from build123d import *

# Parameters (mm, degrees)
SKETCH_1_W          = 250
SKETCH_1_H          = 30
EXTRUDE_1_DEPTH     = 11
SKETCH_4_W          = 15
SKETCH_4_H          = 5
EXTRUDE_2_DEPTH     = 25
CUT_EXTRUDE_2_DEPTH = 251
CUT_EXTRUDE_3_DEPTH = 21
SKETCH_11_W         = 30
SKETCH_11_H         = 10
EXTRUDE_4_DEPTH     = 25
SKETCH_12_R         = 1.6
CUT_EXTRUDE_5_DEPTH = 21
FILLET_1_R          = 10
SKETCH_13_W         = 2
SKETCH_13_H         = 26.2
CUT_EXTRUDE_6_DEPTH = 37
CHAMFER_1_SIZE      = 1


with BuildPart() as part:
    # 草圖1 → 填料-伸長1 (new body)
    with BuildSketch(Plane.XY):
        with Locations((125, 15)):
            Rectangle(SKETCH_1_W, SKETCH_1_H)
    extrude(amount=EXTRUDE_1_DEPTH)

    # 草圖4 → 填料-伸長2 (add)
    with BuildSketch(Plane(origin=(0, 0, 0), x_dir=(-1, 0, 0), z_dir=(0, 0, -1))):
        with Locations((-132.5, 12.5)):
            Rectangle(SKETCH_4_W, SKETCH_4_H)
        with Locations((-132.5, 17.5)):
            Rectangle(SKETCH_4_W, SKETCH_4_H)
        with Locations((-117.5, 17.5)):
            Rectangle(SKETCH_4_W, SKETCH_4_H)
        with Locations((-117.5, 12.5)):
            Rectangle(SKETCH_4_W, SKETCH_4_H)
    extrude(amount=EXTRUDE_2_DEPTH)

    # 草圖5 → 除料-伸長2 (cut, through all)
    with BuildSketch(Plane(origin=(250, 0, 0), x_dir=(0, 0, -1), z_dir=(1, 0, 0))):
        Polygon((-11, 15), (-7, 15), (-7, 18), (-11, 21), align=None)
        Polygon((-7, 12), (-7, 15), (-11, 15), (-11, 9), align=None)
    extrude(amount=-CUT_EXTRUDE_2_DEPTH, mode=Mode.SUBTRACT)

    # 草圖6 → 除料-伸長3 (cut, through all)
    with BuildSketch(Plane.XZ.offset(-10)):
        with BuildLine():
            ThreePointArc((126.6, -12.5), (126.13137085, -11.36862915), (125, -10.9))
            Line((125, -10.9), (125, -12.5))
            Line((125, -12.5), (126.6, -12.5))
        make_face()
        with BuildLine():
            Line((125, -12.5), (125, -10.9))
            ThreePointArc((125, -10.9), (123.86862915, -11.36862915), (123.4, -12.5))
            Line((123.4, -12.5), (125, -12.5))
        make_face()
        with BuildLine():
            Line((126.6, -12.5), (125, -12.5))
            Line((125, -12.5), (125, -14.1))
            ThreePointArc((125, -14.1), (126.13137085, -13.63137085), (126.6, -12.5))
        make_face()
        with BuildLine():
            Line((125, -14.1), (125, -12.5))
            Line((125, -12.5), (123.4, -12.5))
            ThreePointArc((123.4, -12.5), (123.86862915, -13.63137085), (125, -14.1))
        make_face()
    extrude(amount=-CUT_EXTRUDE_3_DEPTH, mode=Mode.SUBTRACT)

    # 草圖11 → 填料-伸長4 (add)
    with BuildSketch(Plane(origin=(0, 0, 0), x_dir=(-1, 0, 0), z_dir=(0, 0, -1))):
        with Locations((-225, 15)):
            Rectangle(SKETCH_11_W, SKETCH_11_H)
    extrude(amount=EXTRUDE_4_DEPTH)

    # 草圖12 → 除料-伸長5 (cut, through all)
    with BuildSketch(Plane(origin=(0, 20, 0), x_dir=(1, 0, 0), z_dir=(0, 1, 0))):
        with Locations((225, 12.5)):
            Circle(SKETCH_12_R)
    extrude(amount=-CUT_EXTRUDE_5_DEPTH, mode=Mode.SUBTRACT)

    # 圓角1
    fillet_1_edges = [part.edges().sort_by_distance(p)[0] for p in [
        (110, 15, -25),
        (140, 15, -25),
        (240, 15, -25),
        (210, 15, -25),
    ]]
    fillet(fillet_1_edges, radius=FILLET_1_R)

    # 草圖13 → 除料-伸長6 (cut, through all)
    with BuildSketch(Plane.XY.offset(11)):
        with Locations((245, 15)):
            Rectangle(SKETCH_13_W, SKETCH_13_H)
    extrude(amount=-CUT_EXTRUDE_6_DEPTH, mode=Mode.SUBTRACT)

    # 導角1
    chamfer_1_edges = [part.edges().sort_by_distance(p)[0] for p in [
        (250, 4.5, 11),
        (125, 30, 11),
        (110, 15, 0),
        (140, 15, 0),
        (125, 10, 0),
        (125, 20, 0),
        (0, 4.5, 11),
        (250, 25.5, 11),
        (250, 10.5, 9),
        (250, 15, 7),
        (250, 19.5, 9),
        (0, 25.5, 11),
        (125, 30, 0),
        (250, 15, 0),
        (125, 0, 0),
        (225, 10, 0),
        (210, 15, 0),
        (0, 15, 0),
        (240, 15, 0),
        (225, 20, 0),
        (125, 0, 11),
        (125, 20, -25),
        (125, 10, -25),
        (0, 30, 5.5),
        (250, 30, 5.5),
        (140, 20, -7.5),
        (110, 20, -7.5),
        (137.071067812, 20, -22.071067812),
        (250, 0, 5.5),
        (112.928932188, 20, -22.071067812),
        (110, 10, -7.5),
        (0, 0, 5.5),
        (140, 10, -7.5),
        (137.071067812, 10, -22.071067812),
        (112.928932188, 10, -22.071067812),
        (225, 10, -25),
        (225, 20, -25),
        (240, 20, -7.5),
        (210, 20, -7.5),
        (237.071067812, 20, -22.071067812),
        (212.928932188, 20, -22.071067812),
        (210, 10, -7.5),
        (240, 10, -7.5),
        (237.071067812, 10, -22.071067812),
        (212.928932188, 10, -22.071067812),
    ]]
    chamfer(chamfer_1_edges, length=CHAMFER_1_SIZE)


solid = part.part
CAD build for the part. Positions are in the model's coordinates, mm. A direction names the side the tool comes from. Round coordinates to 2 decimals unless told otherwise and drop trailing zeros. Order: outer loops, then holes, each group sorted by start corner. A loop starts at its lowest first (then second) coordinate and runs counter-clockwise, first axis right, second up. Notation, with made-up numbers: (30, -13.5) -> (47, -13.5) arc R21 cw to (47, 3.5) -> close; hole circle Ø8 at (68, 15.25). An arc over 180 degrees is marked (long way). Write item = value, one per line. Start each with the question number.
(1) Cut at A-A, the plane z = -8. List the corners of the cut face in (x, y), then the cut area to 3 significant figures.
(2) Pin check, flat tips, straight feed: P1, Ø4, axis at x = 163.5, y = 26.5, coming from the -Z side; P2, Ø1.8, axis at x = 89.5, y = 14.5, coming from the +Z side; P3, Ø9, axis at y = 17, z = -6, coming from the +X side; P4, Ø2.5, axis at x = 225, z = -12.5, coming from the -Y side. Stop position of each tip, or through.
(3) Cut at B-B, the plane x = 61.5. List the corners of the cut face in (y, z).
(4) Probe line 1 (X direction, y = 13.5, z = -12.5); line 2 (Z direction, x = 225, y = 15); line 3 (X direction, y = 22, z = 1.5). List the from-to ranges inside material, lowest first. Write a range as [from, to].
(5) Pull direction X, two halves, no side cores. Call faces 5 (the flat face through (250, 15, 5)), 6 (the conical face through (213.585, 19.826, -21.558)), 7 (the cylindrical face through (112.85, 15.06, -21.99)): released by +X, released by -X, zero draft, split by the parting line, or undercut.
(6) Which spindle directions (+Z, -Z, +X, -X, +Y, -Y) get a long thin tool onto all of the face, cutting with end or side? Do faces 1 (the flat face through (240, 15, -8)), 2 (the flat face through (246, 15, 6)), 3 (the flat face through (123.7, 19.5, 9)), 4 (the flat face through (110, 15, -8)). Say none if no direction does.
Model answer:
q1.outline = (110, 11) -> (111, 10) -> (139, 10) -> (140, 11) -> (140, 19) -> (139, 20) -> (111, 20) -> (110, 19) -> close; (210, 11) -> (211, 10) -> (239, 10) -> (240, 11) -> (240, 19) -> (239, 20) -> (211, 20) -> (210, 19) -> close
q1.area = 596 mm2
q2.P1 = 0
q2.P2 = 7
q2.P3 = 240
q2.P4 = through
q3.outline = (0, 1) -> (1, 0) -> (29, 0) -> (30, 1) -> (30, 10) -> (29, 11) -> (21, 11) -> (18, 7) -> (12, 7) -> (9, 11) -> (1, 11) -> (0, 10) -> close
q4.line_1 = [110, 123.4], [126.6, 140], [210, 223.4], [226.6, 240]
q4.line_2 = [-25, -14.1], [-10.9, 7]
q4.line_3 = [0, 244], [246, 250]
q5.face_5 = released by +X
q5.face_6 = undercut
q5.face_7 = released by -X
q6.face_1 = -Z, +X, +Y, -Y
q6.face_2 = +Z, -Z
q6.face_3 = +Z, +X, -X
q6.face_4 = -Z, -X, +Y, -Y
